Build history of the part. All positions in model axes, mm. A direction names the side the tool comes from. Coordinates: 2 decimals unless noted, no trailing zeros. Order: outer loops, then holes, each group sorted by start corner. A loop starts at its lowest first (then second) coordinate and runs counter-clockwise, first axis right, second up. Notation, with made-up numbers: (78, 47) -> (82, 47) arc R34 ccw to (82, 85) -> close; hole circle Ø5 at (9.5, 73.25). An arc over 180 degrees is marked (long way). Write each question's results on one line, items separated by ' | '.
from build123d import *

# Parameters (mm, degrees)
F1_DEPTH = 19.05
F2_W     = 71.4131370187
F2_H     = 37.0434857905
F3_DEPTH = 38.1
F5_DEPTH = 125.0588758598
F6_W     = 28.5964906216
F6_H     = 18.30278337
F6_H_2   = 9.0631097555
F7_DEPTH = 45.7155236433
F8_R     = 6.3682145367
F9_DEPTH = 125.1160786257


with BuildPart() as f1:
    # F0 (on Front) → F1 (new body)
    with BuildSketch(Plane.XZ):
        with BuildLine():
            Line((62.2737929225, 27.192780748), (-62.2737929225, 27.192780748))
            Line((-62.2737929225, 27.192780748), (-62.2737929225, 27.077514428))
            ThreePointArc((-62.2737929225, 27.077514428), (-43.1270988528, 19.1466940697), (-35.1962784945, 0))
            ThreePointArc((-35.1962784945, 0), (-43.1270988528, -19.1466940697), (-62.2737929225, -27.077514428))
            Line((-62.2737929225, -27.077514428), (-62.2737929225, -27.192780748))
            Line((-62.2737929225, -27.192780748), (62.2737929225, -27.192780748))
            Line((62.2737929225, -27.192780748), (62.2737929225, -27.1347171939))
            ThreePointArc((62.2737929225, -27.1347171939), (35.1390757286, 0), (62.2737929225, 27.1347171939))
            Line((62.2737929225, 27.1347171939), (62.2737929225, 27.192780748))
        make_face()
        with BuildLine():
            ThreePointArc((-35.1962784945, 0), (-43.1270988528, 19.1466940697), (-62.2737929225, 27.077514428))
            Line((-62.2737929225, 27.077514428), (-62.2737929225, 16.5543363838))
            ThreePointArc((-62.2737929225, 16.5543363838), (-50.5681094075, 11.705683515), (-45.7194565387, 0))
            ThreePointArc((-45.7194565387, 0), (-50.5681094075, -11.705683515), (-62.2737929225, -16.5543363838))
            Line((-62.2737929225, -16.5543363838), (-62.2737929225, -27.077514428))
            ThreePointArc((-62.2737929225, -27.077514428), (-43.1270988528, -19.1466940697), (-35.1962784945, 0))
        make_face()
        with BuildLine():
            Line((-62.2737929225, 16.5543363838), (-62.2737929225, 27.077514428))
            ThreePointArc((-62.2737929225, 27.077514428), (-89.3513073505, 0), (-62.2737929225, -27.077514428))
            Line((-62.2737929225, -27.077514428), (-62.2737929225, -16.5543363838))
            ThreePointArc((-62.2737929225, -16.5543363838), (-78.8281293062, 0), (-62.2737929225, 16.5543363838))
        make_face()
        with BuildLine():
            Line((62.2737929225, 17.6446747149), (62.2737929225, 27.1347171939))
            ThreePointArc((62.2737929225, 27.1347171939), (35.1390757286, 0), (62.2737929225, -27.1347171939))
            Line((62.2737929225, -27.1347171939), (62.2737929225, -17.6446747149))
            ThreePointArc((62.2737929225, -17.6446747149), (44.6291182076, 0), (62.2737929225, 17.6446747149))
        make_face()
        with BuildLine():
            ThreePointArc((89.4085101164, 0), (81.4609354559, 19.1871425334), (62.2737929225, 27.1347171939))
            Line((62.2737929225, 27.1347171939), (62.2737929225, 17.6446747149))
            ThreePointArc((62.2737929225, 17.6446747149), (74.7504620652, 12.4766691427), (79.9184676374, 0))
            ThreePointArc((79.9184676374, 0), (74.7504620652, -12.4766691427), (62.2737929225, -17.6446747149))
            Line((62.2737929225, -17.6446747149), (62.2737929225, -27.1347171939))
            ThreePointArc((62.2737929225, -27.1347171939), (81.4609354559, -19.1871425334), (89.4085101164, 0))
        make_face()
    extrude(amount=F1_DEPTH)

    # F2 (on face) → F3 (join)
    with BuildSketch(Plane.XZ.offset(19.05)):
        Rectangle(F2_W, F2_H)
    extrude(amount=F3_DEPTH)

    # F4 (on face) → F5 (cut, through all)
    with BuildSketch(Plane.YZ.offset(35.7065685093)):
        with BuildLine():
            ThreePointArc((-42.3361994326, -18.5217428952), (-56.4047103889, 0), (-42.3361994326, 18.5217428952))
            Line((-42.3361994326, 18.5217428952), (-57.15, 18.5217428952))
            Line((-57.15, 18.5217428952), (-57.15, -18.5217428952))
            Line((-57.15, -18.5217428952), (-42.3361994326, -18.5217428952))
        make_face()
    extrude(amount=-F5_DEPTH, mode=Mode.SUBTRACT)

    # F6 (on face) → F7 (cut, through all)
    with BuildSketch(Plane(origin=(0, 0, -18.5217428952), x_dir=(1, 0, 0), z_dir=(0, 0, -1))):
        with Locations((0, 51.4875911176)):
            Rectangle(F6_W, F6_H)
        with Locations((0, 37.8046445549)):
            Rectangle(F6_W, F6_H_2)
        with BuildLine():
            Line((14.2982453108, 33.2730896771), (-14.2982453108, 33.2730896771))
            ThreePointArc((-14.2982453108, 33.2730896771), (0, 21.3200343577), (14.2982453108, 33.2730896771))
        make_face()
    extrude(amount=-F7_DEPTH, mode=Mode.SUBTRACT)

    # F8 (on face) → F9 (cut, through all)
    with BuildSketch(Plane(origin=(-35.7065685093, 0, 0), x_dir=(0, -1, 0), z_dir=(-1, 0, 0))):
        with Locations((43.9249239862, 0)):
            Circle(F8_R)
    extrude(amount=-F9_DEPTH, mode=Mode.SUBTRACT)


solid = f1.part
Item 1: Drill centre lines: line 1 (X direction, y = -38.5, z = 6); line 2 (X direction, y = -13, z = -13); line 3 (X direction, y = -8.5, z = -4). Where is each one in solid material? Low to high. Write a range as from..to.
Answer:
line 1: x = -35.71..-14.3, 14.3..35.71 | line 2: x = -86.03..-72.52, -52.02..50.34, 74.2..86.09 | line 3: x = -89.05..-78.34, -46.21..45.09, 79.46..89.11
Item 2: Slice it at D-D, the plane y = -40.5. List the corners of the cut face in (x, z).
Answer:
outline: (-35.71, -18.52) -> (-14.3, -18.52) -> (-14.3, -5.37) -> (-35.71, -5.37) -> close; (-35.71, 5.37) -> (-14.3, 5.37) -> (-14.3, 18.52) -> (-35.71, 18.52) -> close; (14.3, -18.52) -> (35.71, -18.52) -> (35.71, -5.37) -> (14.3, -5.37) -> close; (14.3, 5.37) -> (35.71, 5.37) -> (35.71, 18.52) -> (14.3, 18.52) -> close
Item 3: Pin check, flat tips, straight feed: pin 1 (10 mm diameter, centred on y = -21, z = -18.5, fed in from -X); pin 2 (12 mm diameter, centred on x = -32, z = 13, fed in from -Y); pin 3 (11.5 mm diameter, centred on x = -12, y = -35, fed in from +Z). Stop position of each tip, or through.
Answer:
pin 1: stops at x = -85.51 | pin 2: stops at y = -55.09 | pin 3: stops at z = 18.52
Item 4: Tool access for faces 1 (the flat face through (35.707, -33, 0)), 2 (the flat face through (0, -20, -18.522)), 3 (the flat face through (0, -20, 18.522)), 4 (the flat face through (-35.707, -33, 0)): list every direction of +Z, -Z, +X, -X, +Y, -Y with a clear straight run to the whole face (end or side of a thin tool).
Answer:
face 1: +Z, -Z, +X, -Y | face 2: -Z, +X, -X, -Y | face 3: +Z, +X, -X, -Y | face 4: +Z, -Z, -X, -Y
Item 5: Slice it at C-C, the plane x = 71. List the corners of the cut face in (y, z).
Answer:
outline: (-19.05, -25.69) -> (0, -25.69) -> (0, -15.34) -> (-19.05, -15.34) -> close; (-19.05, 15.34) -> (0, 15.34) -> (0, 25.69) -> (-19.05, 25.69) -> close
Item 6: Slice it at B-B, the plane z = 13. List the corners of the cut face in (x, y), and give its area (3 significant figures).
Answer:
outline: (-86.03, -19.05) -> (-72.52, -19.05) -> (-72.52, 0) -> (-86.03, 0) -> close; (-52.02, -19.05) -> (-35.71, -19.05) -> (-35.71, -51.34) -> (-14.3, -51.34) -> (-14.3, -33.27) arc R14.53 cw to (14.3, -33.27) -> (14.3, -51.34) -> (35.71, -51.34) -> (35.71, -19.05) -> (50.34, -19.05) -> (50.34, 0) -> (-52.02, 0) -> close; (74.2, -19.05) -> (86.09, -19.05) -> (86.09, 0) -> (74.2, 0) -> close | area: 3,970 mm^2
Item 7: Pull direction Z, two halves, no side cores. Call faces 5 (the flat face through (-1, -9, -27.193)), 6 (the cylindrical face through (25.15, -56.4, -0.35)), 7 (the cylindrical face through (-25.152, -37.563, 0.28)): released by +Z, released by -Z, zero draft, split by the parting line, or undercut.
Answer:
face 5: released by -Z | face 6: split by the parting line | face 7: undercut
Item 8: Slice it at A-A, the plane y = -8. List the corners of the cut face in (x, z).
Answer:
outline: (-62.27, -27.19) -> (62.27, -27.19) -> (62.27, -27.13) arc R27.13 ccw to (62.27, 27.13) -> (62.27, 27.19) -> (-62.27, 27.19) -> (-62.27, 27.08) arc R27.08 ccw to (-62.27, -27.08) -> close; hole circle Ø33.11 at (-62.27, 0); hole circle Ø35.29 at (62.27, 0)
